The model under review builds one solid part; all positions refer to its coordinate system, in mm. Give positions to 0.01 mm unless a question says otherwise; leave off trailing zeros. Write each loop counter-clockwise with the first axis right and the second up, starting at its lowest first coordinate (ties: lowest second). Pieces come first, ordered by that corner, then holes.
from build123d import *

# Parameters (mm, degrees)
SKETCH_1_R      = 80
SKETCH_1_R_2    = 6.269952148
SKETCH_1_R_3    = 2
SKETCH_1_R_4    = 2.5
SKETCH_1_R_5    = 2.214537903
SKETCH_1_R_6    = 2.039490197
SKETCH_1_W      = 41
SKETCH_1_H      = 21
EXTRUDE_1_DEPTH = 3


with BuildPart() as part:
    # ｽｹｯﾁ1 → ﾎﾞｽ - 押し出し1 (new body)
    with BuildSketch(Plane(origin=(0, 0, 0), x_dir=(0, 0, -1), z_dir=(1, 0, 0))):
        with Locations((-2426.873769578, 1479.495473195)):
            Circle(SKETCH_1_R)
        with Locations((-2388.873769578, 1479.495473195)):
            Circle(SKETCH_1_R_2, mode=Mode.SUBTRACT)
        with Locations((-2412.323769578, 1484.395473195)):
            Circle(SKETCH_1_R_3, mode=Mode.SUBTRACT)
        with Locations((-2412.323769578, 1474.595473195)):
            Circle(SKETCH_1_R_3, mode=Mode.SUBTRACT)
        with Locations((-2461.323769578, 1484.395473195)):
            Circle(SKETCH_1_R_3, mode=Mode.SUBTRACT)
        with Locations((-2461.323769578, 1474.595473195)):
            Circle(SKETCH_1_R_3, mode=Mode.SUBTRACT)
        with Locations((-2492.495547842, 1505.835219157)):
            Circle(SKETCH_1_R_4, mode=Mode.SUBTRACT)
        with Locations((-2482.495547842, 1523.155727232)):
            Circle(SKETCH_1_R_3, mode=Mode.SUBTRACT)
        with Locations((-2436.873769578, 1549.495473195)):
            Circle(SKETCH_1_R_4, mode=Mode.SUBTRACT)
        with Locations((-2416.873769578, 1549.495473195)):
            Circle(SKETCH_1_R_3, mode=Mode.SUBTRACT)
        with Locations((-2371.251991313, 1523.155727232)):
            Circle(SKETCH_1_R_5, mode=Mode.SUBTRACT)
        with Locations((-2361.251991313, 1505.835219157)):
            Circle(SKETCH_1_R_3, mode=Mode.SUBTRACT)
        with Locations((-2361.251991313, 1453.155727232)):
            Circle(SKETCH_1_R_4, mode=Mode.SUBTRACT)
        with Locations((-2371.251991313, 1435.835219157)):
            Circle(SKETCH_1_R_3, mode=Mode.SUBTRACT)
        with Locations((-2416.873769578, 1409.495473195)):
            Circle(SKETCH_1_R_4, mode=Mode.SUBTRACT)
        with Locations((-2436.873769578, 1409.495473195)):
            Circle(SKETCH_1_R_3, mode=Mode.SUBTRACT)
        with Locations((-2482.495547842, 1435.835219157)):
            Circle(SKETCH_1_R_4, mode=Mode.SUBTRACT)
        with Locations((-2492.495547842, 1453.155727232)):
            Circle(SKETCH_1_R_6, mode=Mode.SUBTRACT)
        with Locations((-2436.823769578, 1479.495473195)):
            Rectangle(SKETCH_1_W, SKETCH_1_H, mode=Mode.SUBTRACT)
    extrude(amount=EXTRUDE_1_DEPTH)


solid = part.part
1) Consider section C-C, the plane y = 1539. Give the boundary of the cut face in (x, z), then the cut area to 3 significant figures.
2) Consider section A-A, the plane x = 1.1. State how many separate pieces and enclosed holes the cut face has, then the cut area to 3 significant figures.
3) Insertion check: pin 1 (1.5 mm diameter, centred on x = 0.5, y = 1516, fed in from +Z); pin 2 (0.9 mm diameter, centred on x = 2, y = 1484, fed in from +Z). Each pin has a flat end and moves straight along its axis. Give the tip position at first contact, or say it passes through.
4) To check wall thickness, follow probe 1 along Y at (x, z) = (0.7, 2411); probe 2 along Z at (x, y) = (0.65, 1486); probe 3 along Y at (x, z) = (0.25, 2362). State the ranges of each line that lie inside material, in increasing order.
5) Consider section B-B, the plane z = 2377.5. Give the boundary of the cut face in (x, y).
Answer block:
1. outline: (0, 2373.4) - (3, 2373.4) - (3, 2480.35) - (0, 2480.35) - close
1. area: 321 mm2
2. separate pieces: 1
2. enclosed holes: 18
2. area: 18,900 mm2
3. pin 1: stops at z = 2498.44
3. pin 2: stops at z = 2506.77
4. probe 1: y = 1401.09 to 1473.1, 1476.09 to 1482.9, 1485.89 to 1557.9
4. probe 2: z = 2347.14 to 2411.13, 2413.52 to 2416.32, 2457.32 to 2460.13, 2462.52 to 2506.61
4. probe 3: y = 1432.68 to 1450.77, 1455.54 to 1503.98, 1507.69 to 1526.31
5. outline: (0, 1416.55) - (3, 1416.55) - (3, 1542.44) - (0, 1542.44) - close
